```python
from build123d import *

# Parameters (mm, degrees)
FILLET_1_R             = 1
HOLE_WIZARD_M8_1_D     = 6.8
HOLE_WIZARD_M8_1_DEPTH = 20
HOLE_WIZARD_M8_1_TIP   = 2.042926105
CUT_EXTRUDE_1_DEPTH    = 83.012194246


with BuildPart() as part:
    # 草图1 → 旋转1 (revolve)
    with BuildSketch(Plane.XY, mode=Mode.PRIVATE) as revolve_1_sk:
        Polygon((0, 0), (0, 80), (-6, 80), (-6, 6), (-25, 6), (-25, 0), align=None)
    revolve(revolve_1_sk.sketch.rotate(Axis((0, 0, 0), (0, 1, 0)), 270), axis=Axis((0, 0, 0), (0, 1, 0)))

    # 圆角1
    fillet_1_edges = [part.edges().sort_by_distance(p)[0] for p in [
        (0, 6, 25),
    ]]
    fillet(fillet_1_edges, radius=FILLET_1_R)

    # M8 螺纹槽口的螺纹槽口钻头1
    with Locations(Plane(origin=(0, 80, 0), x_dir=(1, 0, 0), z_dir=(0, 1, 0))):
        with Locations((0, 0)):
            Hole(HOLE_WIZARD_M8_1_D / 2, depth=HOLE_WIZARD_M8_1_DEPTH)
            with Locations((0, 0, -(HOLE_WIZARD_M8_1_DEPTH + HOLE_WIZARD_M8_1_TIP / 2))):  # 118° drill point
                Cone(0, HOLE_WIZARD_M8_1_D / 2, HOLE_WIZARD_M8_1_TIP, mode=Mode.SUBTRACT)

    # 草图5 → 切除-拉伸1 (cut, through all)
    with BuildSketch(Plane(origin=(0, 6, 0), x_dir=(1, 0, 0), z_dir=(0, 1, 0))):
        with BuildLine():
            Line((12.121320344, -7.878679656), (22.727922061, -18.485281374))
            ThreePointArc((22.727922061, -18.485281374), (22.727922061, -22.727922061), (18.485281374, -22.727922061))
            Line((18.485281374, -22.727922061), (7.878679656, -12.121320344))
            ThreePointArc((7.878679656, -12.121320344), (7.878679656, -7.878679656), (12.121320344, -7.878679656))
        make_face()
        with BuildLine():
            Line((-7.878679656, -12.121320344), (-18.485281374, -22.727922061))
            ThreePointArc((-18.485281374, -22.727922061), (-22.727922061, -22.727922061), (-22.727922061, -18.485281374))
            Line((-22.727922061, -18.485281374), (-12.121320344, -7.878679656))
            ThreePointArc((-12.121320344, -7.878679656), (-7.878679656, -7.878679656), (-7.878679656, -12.121320344))
        make_face()
        with BuildLine():
            Line((-12.121320344, 7.878679656), (-22.727922061, 18.485281374))
            ThreePointArc((-22.727922061, 18.485281374), (-22.727922061, 22.727922061), (-18.485281374, 22.727922061))
            Line((-18.485281374, 22.727922061), (-7.878679656, 12.121320344))
            ThreePointArc((-7.878679656, 12.121320344), (-7.878679656, 7.878679656), (-12.121320344, 7.878679656))
        make_face()
        with BuildLine():
            Line((7.878679656, 12.121320344), (18.485281374, 22.727922061))
            ThreePointArc((18.485281374, 22.727922061), (22.727922061, 22.727922061), (22.727922061, 18.485281374))
            Line((22.727922061, 18.485281374), (12.121320344, 7.878679656))
            ThreePointArc((12.121320344, 7.878679656), (7.878679656, 7.878679656), (7.878679656, 12.121320344))
        make_face()
    extrude(amount=-CUT_EXTRUDE_1_DEPTH, mode=Mode.SUBTRACT)


solid = part.part
```
The listing builds one solid part. Answer for the finished solid, in the listing's coordinates (mm). A direction names the side the tool comes from. Round coordinates to 2 decimals unless told otherwise and drop trailing zeros. Loops run counter-clockwise (first coordinate to the right, second up) from the corner with the lowest first, then second, coordinate; pieces in that order, holes last. Notation, with made-up numbers: (-21, 4.5) - (37, 4.5) arc R26 ccw to (37, 25.5) - close; hole circle Ø4 at (32, 45). An arc over 180 degrees is marked (long way). Return JSON: item names as keys, results as strings. Group by question number.
1. Consider probe 1 along Y at (x, z) = (18, -4); probe 2 along Z at (x, y) = (4.5, 15); probe 3 along Z at (x, y) = (4, 28.5). Determine where each line is inside the solid, lowest interval first.
2. The part is cut by section B-B on y = 21.5. Determine the outline of the cut face in (x, z).
3. Each of these flat-tipped pins is pushed along its axis until it touches: P1, Ø10, axis at y = 66.5, z = 5, coming from the -X side; P2, Ø5, axis at x = -8, z = -11, coming from the +Y side; P3, Ø6, axis at x = 4, y = 38, coming from the +Z side. Where does it stop, or does it pass through?
4. The part is cut by section A-A on y = 63.5. Determine the outline of the cut face in (x, z), then the cut area to 3 significant figures.
5. The part is cut by section C-C on z = -13. State how many separate pieces and enclosed holes the cut face has, then the cut area to 3 significant figures.
6. Which of the six approach directions +Z, -Z, +X, -X, +Y, -Y give full straight-line access (tool end or side, diameter ignored) to faces 5 (the flat face through (5, 6, 5)), 6 (the flat face through (0, 0, 0)), 7 (the flat face through (-11.71, 3.04, -15.95))?
7. The mould has two halves that part along X. Classify faces 1 (the cylindrical face through (0.74, 69.86, 3.32)), 2 (the cylindrical face through (0, 2, 25)), 3 (the cylindrical face through (25, 2, 0)), 4 (the flat face through (3, 80, 3)): pulls with the +X half, pulls with the -X half, needs draft (parallel to the pull), parting line crosses it, or undercut.
Resolved:
{
 "1": {"probe 1": "y = 0 to 6", "probe 2": "z = -3.97 to 3.97", "probe 3": "z = -4.47 to 4.47"},
 "2": {"outline": "circle Ø12 at (0, 0)"},
 "3": {"P1": "stops at x = -6", "P2": "stops at y = 6", "P3": "stops at z = 5.92"},
 "4": {"outline": "circle Ø12 at (0, 0); hole circle Ø6.8 at (0, 0)", "area": "76.8 mm²"},
 "5": {"separate pieces": "3", "enclosed holes": "0", "area": "154 mm²"},
 "6": {"face 5": "+Y", "face 6": "+Z, -Z, +X, -X, -Y", "face 7": "+Y, -Y"},
 "7": {"face 1": "undercut", "face 2": "parting line crosses it", "face 3": "pulls with the +X half", "face 4": "needs draft"}
}
